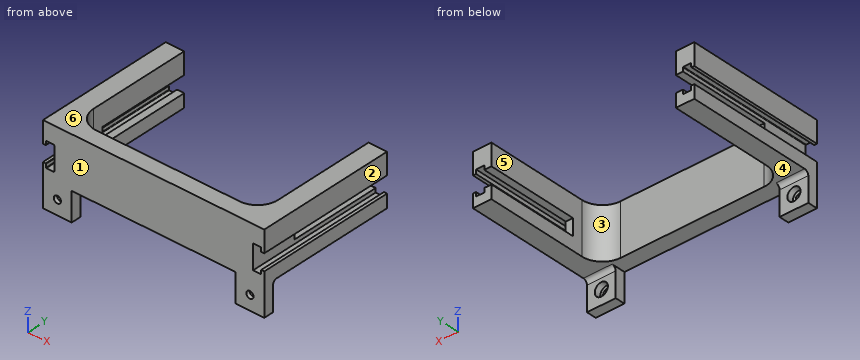
```python
from build123d import *

# Parameters (mm, degrees)
BOSS_EXTRUDE1_DEPTH = 15
CUT_EXTRUDE1_DEPTH  = 67.82
SKETCH3_W           = 3.5
SKETCH3_H           = 8
CUT_EXTRUDE2_DEPTH  = 45
FILLET1_R           = 0.25
BOSS_EXTRUDE2_DEPTH = 7
BOSS_EXTRUDE3_DEPTH = 3
FILLET2_R           = 10
SKETCH12_W          = 14
SKETCH12_H          = 4.82
BOSS_EXTRUDE4_DEPTH = 14
FILLET3_R           = 2


with BuildPart() as part:
    # Sketch1 → Boss-Extrude1 (new body)
    with BuildSketch(Plane.XY):
        Polygon((-54, 0), (54, 0), (54, 67.82), (45, 67.82), (45, 7.82), (-45, 7.82), (-45, 67.82), (-54, 67.82), align=None)
    extrude(amount=-BOSS_EXTRUDE1_DEPTH)

    # Sketch2 → Cut-Extrude1 (cut)
    with BuildSketch(Plane(origin=(0, 67.82, 0), x_dir=(1, 0, 0), z_dir=(0, 1, 0))):
        Polygon((-54, 11.5), (-52.5, 11.5), (-52.5, 13.5), (-48.5, 13.5), (-48.5, 1.5), (-52.5, 1.5), (-52.5, 3.5), (-54, 3.5), align=None)
    cut_extrude1 = extrude(amount=-CUT_EXTRUDE1_DEPTH, mode=Mode.SUBTRACT)

    # Sketch3 → Cut-Extrude2 (cut)
    with BuildSketch(Plane(origin=(0, 67.82, 0), x_dir=(1, 0, 0), z_dir=(0, 1, 0))):
        with Locations((-46.75, 7.5)):
            Rectangle(SKETCH3_W, SKETCH3_H)
    cut_extrude2 = extrude(amount=-CUT_EXTRUDE2_DEPTH, mode=Mode.SUBTRACT)

    # Fillet1
    fillet1_edges = [part.edges().sort_by_distance(p)[0] for p in [
        (-52.5, 33.91, -3.5),
        (-52.5, 33.91, -1.5),
        (-48.5, 33.91, -1.5),
        (-48.5, 33.91, -13.5),
        (-52.5, 33.91, -13.5),
        (-52.5, 33.91, -11.5),
    ]]
    fillet(fillet1_edges, radius=FILLET1_R)

    # Mirror1: Cut-Extrude1 across plane
    add(cut_extrude1.mirror(Plane(origin=(0, 0, 0), x_dir=(0, 0, 1), z_dir=(1, 0, 0))), mode=Mode.SUBTRACT)

    # Mirror2: Cut-Extrude2 across plane
    add(cut_extrude2.mirror(Plane(origin=(0, 0, 0), x_dir=(0, 0, 1), z_dir=(1, 0, 0))), mode=Mode.SUBTRACT)

    # Sketch7 → Boss-Extrude2 (add)
    with BuildSketch(Plane.XY):
        Polygon((-54, 67.82), (-54, 0), (54, 0), (54, 67.82), (45, 67.82), (45, 7.82), (-45, 7.82), (-45, 67.82), align=None)
    extrude(amount=BOSS_EXTRUDE2_DEPTH)

    # Sketch11 → Boss-Extrude3 (add)
    with BuildSketch(Plane(origin=(0, 0, -15), x_dir=(-1, 0, 0), z_dir=(0, 0, -1))):
        Polygon((54, 0), (54, 67.82), (45, 67.82), (45, 7.82), (-45, 7.82), (-45, 67.82), (-54, 67.82), (-54, 0), align=None)
    extrude(amount=BOSS_EXTRUDE3_DEPTH)

    # Fillet2
    fillet2_edges = [part.edges().sort_by_distance(p)[0] for p in [
        (-45, 7.82, -5.5),
        (45, 7.82, -5.5),
    ]]
    fillet(fillet2_edges, radius=FILLET2_R)

    # Sketch12 → Boss-Extrude4 (add)
    with BuildSketch(Plane.XY.offset(-18)):
        with Locations((-47, 2.41)):
            Rectangle(SKETCH12_W, SKETCH12_H)
        with Locations((47, 2.41)):
            Rectangle(SKETCH12_W, SKETCH12_H)
    extrude(amount=-BOSS_EXTRUDE4_DEPTH)

    # Sketch13 → Cut-Revolve1 (revolve, cut)
    with BuildSketch(Plane.ZY.offset(47)):
        Polygon((-25, 4.82), (-25, 0), (-23.26, 0), (-23.26, 1.82), (-21.8, 1.82), (-21.8, 4.82), align=None)
    cut_revolve1 = revolve(axis=Axis((-47, 4.82, -25), (0, -1, 0)), mode=Mode.SUBTRACT)

    # Mirror3: Cut-Revolve1 across plane
    add(cut_revolve1.mirror(Plane(origin=(0, 0, 0), x_dir=(0, 0, 1), z_dir=(1, 0, 0))), mode=Mode.SUBTRACT)

    # Fillet3
    fillet3_edges = [part.edges().sort_by_distance(p)[0] for p in [
        (-47, 4.82, -18),
        (47, 4.82, -18),
    ]]
    fillet(fillet3_edges, radius=FILLET3_R)


solid = part.part
```
Part model, mm, in its own coordinate system. Face numbers are marked on the shaded views. A direction names the side the tool comes from. Give positions to 0.01 mm unless a question says otherwise; leave off trailing zeros. Write each loop counter-clockwise with the first axis right and the second up, starting at its lowest first coordinate (ties: lowest second). Pieces come first, ordered by that corner, then holes. Notation, with made-up numbers: (-11, -32) -> (0, -32) arc R14 ccw to (0, -12) -> close; hole circle Ø2 at (86, 40.25). An arc over 180 degrees is marked (long way). Put each result on its own line as item: value. Start each with the question number.
Item 1: Pin check, flat tips, straight feed: pin 1 Ø1.8 at (x, z) = (-46, -7) entering from +Y; pin 2 Ø1.9 at (x, z) = (-47, -25) entering from +Y; pin 3 Ø4 at (y, z) = (56, -5) entering from +X; pin 4 Ø12 at (x, z) = (-37.5, -11.5) entering from +Y. Stop position of each tip, or through.
Item 2: Which spindle directions (+Z, -Z, +X, -X, +Y, -Y) get a long thin tool onto all of the face, cutting with end or side? Do the marked faces 4, 5 and 6. Say none if no direction does.
Item 3: Wall check: L1, parallel to X at y = 3.85, z = -25; L2, parallel to X at y = 1.15, z = -25; L3, parallel to Z at x = -47, y = 0.5. Give the ranges that are in metal, low to high. Write a range as [from, to].
Item 4: Cut at B-B (x = 47). List the corners of the cut face in (y, z).
Item 5: Cut at C-C (z = -9.5). List the corners of the cut face in (x, y).
Item 6: Pull direction X, two halves, no side cores. Call the marked faces 1, 2 and 3: pulls with the +X half, pulls with the -X half, needs draft (parallel to the pull), parting line crosses it, or undercut.
Item 7: Cut at D-D (x = -2). List the corners of the cut face in (y, z).
Item 8: Cut at A-A (z = -25). List the corners of the cut face in (x, y), then the cut area to 3 significant figures.
Answer list:
1. pin 1: stops at y = 22.82
1. pin 2: passes through
1. pin 3: stops at x = 54
1. pin 4: stops at y = 12.55
2. face 4: -Z, +Y
2. face 5: +Z, -Z, +Y
2. face 6: +Z, +X, -X, +Y, -Y
3. L1: x = [-54, -50.2], [-43.8, -40], [40, 43.8], [50.2, 54]
3. L2: x = [-54, -48.74], [-45.26, -40], [40, 45.26], [48.74, 54]
3. L3: z = [-32, -26.74], [-23.26, 7]
4. outline: (0, -32) -> (4.82, -32) -> (4.82, -28.2) -> (1.82, -28.2) -> (1.82, -26.74) -> (0, -26.74) -> close; (0, -23.26) -> (1.82, -23.26) -> (1.82, -21.8) -> (4.82, -21.8) -> (4.82, -20) arc R2 cw to (6.82, -18) -> (67.82, -18) -> (67.82, -11.5) -> (22.82, -11.5) -> (22.82, -3.5) -> (67.82, -3.5) -> (67.82, 7) -> (0, 7) -> close
5. outline: (-48.5, 0) -> (48.5, 0) -> (48.5, 22.82) -> (45, 22.82) -> (45, 17.82) arc R10 cw to (35, 7.82) -> (-35, 7.82) arc R10 cw to (-45, 17.82) -> (-45, 22.82) -> (-48.5, 22.82) -> close
6. face 1: needs draft
6. face 2: pulls with the +X half
6. face 3: undercut
7. outline: (0, -18) -> (7.82, -18) -> (7.82, 7) -> (0, 7) -> close
8. outline: (-54, 0) -> (-48.74, 0) -> (-48.74, 1.82) -> (-50.2, 1.82) -> (-50.2, 4.82) -> (-54, 4.82) -> close; (-45.26, 0) -> (-40, 0) -> (-40, 4.82) -> (-43.8, 4.82) -> (-43.8, 1.82) -> (-45.26, 1.82) -> close; (40, 0) -> (45.26, 0) -> (45.26, 1.82) -> (43.8, 1.82) -> (43.8, 4.82) -> (40, 4.82) -> close; (48.74, 0) -> (54, 0) -> (54, 4.82) -> (50.2, 4.82) -> (50.2, 1.82) -> (48.74, 1.82) -> close
8. area: 83.9 mm2
